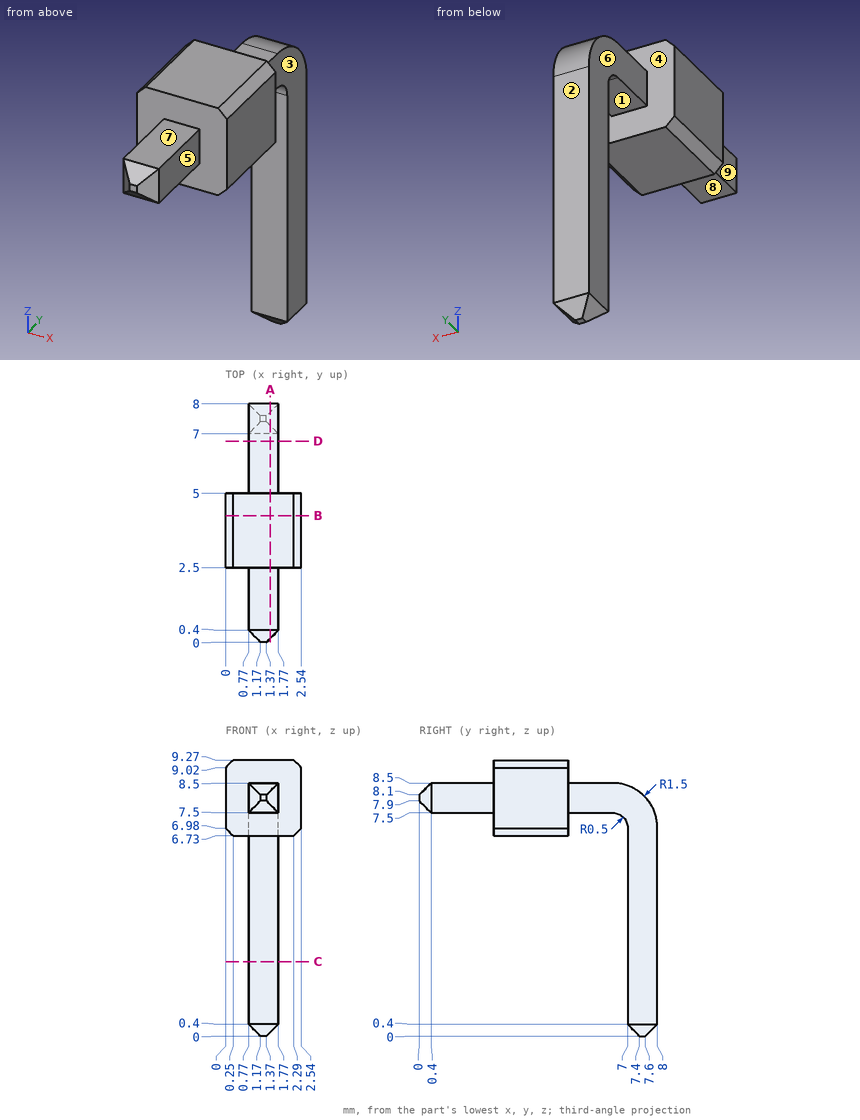
Here's the drawing with two shaded views (mm, measured from the low corner). I have some questions. A direction names the side the tool comes from. Coordinates: 2 decimals unless noted, no trailing zeros. Order: outer loops, then holes, each group sorted by start corner. A loop starts at its lowest first (then second) coordinate and runs counter-clockwise, first axis right, second up.
Item 1: For the marked faces 5, 6, 7, 8 and 9, which set-ups out of +Z, -Z, +X, -X, +Y, -Y let a thin tool reach every point of the face, with its end or its side?
Result sheet:
face 5: +Z, -Z, +X, -Y
face 6: +Z, -Z, -X, +Y
face 7: +Z, +X, -X, -Y
face 8: -Z, +X, -X, -Y
face 9: +Z, -Z, -X, -Y
Item 2: If we section it at C-C on z = 2.5: List the corners of the cut face in (x, y) for me, plus the area to 3 significant figures.
Result sheet:
outline: (0.77, 7) - (1.77, 7) - (1.77, 8) - (0.77, 8) - close
area: 1.00 mm2
Item 3: If we section it at B-B on y = 4.25: List the corners of the cut face in (x, z) for me.
Result sheet:
outline: (0, 6.98) - (0.25, 6.73) - (2.29, 6.73) - (2.54, 6.98) - (2.54, 9.02) - (2.29, 9.27) - (0.25, 9.27) - (0, 9.02) - close
Item 4: I need wall thicknesses on line 1 (Y direction, x = 1.25, z = 4); line 2 (Z direction, x = 1.9, y = 4); line 3 (Z direction, x = 1.3, y = 6). Which ranges of each line are inside material? Lowest first, please.
Result sheet:
line 1: y = 7 to 8
line 2: z = 6.73 to 9.27
line 3: z = 7.5 to 8.5
Item 5: If we mould it in two halves opening along Y, with no side actions, what happens to the marked faces 1, 2, 3 and 4? For each: +Y half, -Y half, draft (parallel to the pull), parting line (faces both ways), or undercut.
Result sheet:
face 1: undercut
face 2: +Y half
face 3: draft
face 4: undercut
Item 6: For P1, Ø1.1, axis at x = 1, y = 5.5, coming from the -Z side; P2, Ø1.1, axis at x = 1.5, y = 1.5, coming from the +Z side; P3, Ø0.5, axis at x = 1.5, y = 1.5, coming from the -Z side; P4, Ø0.9, axis at y = 6.5, z = 3, coming from the -X side, each with a flat end and sliding along its axis, tell me the tip position at first contact or that it passes through.
Result sheet:
P1: stops at z = 6.73
P2: stops at z = 8.5
P3: stops at z = 7.5
P4: passes through
Item 7: If we section it at D-D on y = 6.75: List the corners of the cut face in (x, z) for me.
Result sheet:
outline: (0.77, 7.43) - (1.77, 7.43) - (1.77, 8.48) - (0.77, 8.48) - close
Item 8: If we section it at A-A on x = 1.5: List the corners of the cut face in (y, z) for me, plus the area to 3 significant figures.
Result sheet:
outline: (0.13, 7.77) - (0.4, 7.5) - (2.5, 7.5) - (2.5, 6.73) - (5, 6.73) - (5, 7.5) - (6.5, 7.5) arc R0.5 cw to (7, 7) - (7, 0.4) - (7.27, 0.13) - (7.73, 0.13) - (8, 0.4) - (8, 7) arc R1.5 ccw to (6.5, 8.5) - (5, 8.5) - (5, 9.27) - (2.5, 9.27) - (2.5, 8.5) - (0.4, 8.5) - (0.13, 8.23) - close
area: 18.5 mm2
